Design review of the part built by this model. Coordinates are the model's own, in mm. A direction names the side the tool comes from. Coordinates: 2 decimals unless noted, no trailing zeros. Write each loop counter-clockwise with the first axis right and the second up, starting at its lowest first coordinate (ties: lowest second). Pieces come first, ordered by that corner, then holes. Notation, with made-up numbers: (-35, 1.25) -> (21, 1.25) arc R19 ccw to (21, 38.25) -> close; hole circle Ø6 at (-24, 42). An arc over 180 degrees is marked (long way). Write item = value, one per line. Start each with the question number.
```python
from build123d import *

# Parameters (mm, degrees)
SKETCH1_W                  = 30
SKETCH1_H                  = 30
SKETCH1_R                  = 1.6
SKETCH1_W_2                = 81.01
SKETCH1_H_2                = 12
BOSS_EXTRUDE1_DEPTH        = 6
SKETCH1_3_W                = 30
SKETCH1_3_H                = 30
SKETCH1_3_R                = 1.6
BOSS_EXTRUDE2_DEPTH        = 22.33
CUT_EXTRUDE1_DEPTH         = 88.671255266
SKETCH3_R                  = 2.55
CUT_EXTRUDE2_DEPTH         = 8
CUT_EXTRUDE3_DEPTH         = 4.5
SKETCH6_R                  = 5
CUT_EXTRUDE5_DEPTH         = 8.6
SKETCH7_R                  = 1.6
CUT_EXTRUDE6_DEPTH         = 112.183402538
SKETCH8_R                  = 2.85
CUT_EXTRUDE7_DEPTH         = 18
BOSS_EXTRUDE3_START        = 2.43
SKETCH9_R                  = 3.4
SKETCH9_R_2                = 2.55
BOSS_EXTRUDE3_DEPTH        = 2.43
CHAMFER1_SIZE              = 1.2
FILLET3_R                  = 4
CHAMFER2_SIZE              = 0.8
BOSS_EXTRUDE6_DEPTH        = 14
CUT_EXTRUDE10_REACH        = 116.661
SKETCH17_R                 = 1.1
FILLET5_R                  = 2
CUT_EXTRUDE11_DEPTH        = 3
CHAMFER3_SIZE              = 0.8
LPATTERN2_COUNT            = 3
LPATTERN2_PITCH            = 25
CHAMFER3_OF_LPATTERN2_SIZE = 0.8


with BuildPart() as part:
    # Sketch1 → Boss-Extrude1 (new body)
    # profile 1 of 2: a face of its own
    with BuildSketch(Plane.XY):
        with Locations((10, 10)):
            Rectangle(SKETCH1_W, SKETCH1_H)
        with Locations((20, 0)):
            Circle(SKETCH1_R, mode=Mode.SUBTRACT)
        with Locations((20, 20)):
            Circle(SKETCH1_R, mode=Mode.SUBTRACT)
        with Locations((0, 20)):
            Circle(SKETCH1_R, mode=Mode.SUBTRACT)
        Circle(SKETCH1_R, mode=Mode.SUBTRACT)
    # profile 2 of 2: a face of its own
    with BuildSketch(Plane.XY):
        with Locations((65.505, 10)):
            Rectangle(SKETCH1_W_2, SKETCH1_H_2)
    extrude(amount=BOSS_EXTRUDE1_DEPTH)

    # Sketch1<3> → Boss-Extrude2 (add)
    with BuildSketch(Plane.XY):
        with Locations((10, 10)):
            Rectangle(SKETCH1_3_W, SKETCH1_3_H)
        with Locations((20, 0)):
            Circle(SKETCH1_3_R, mode=Mode.SUBTRACT)
        with Locations((20, 20)):
            Circle(SKETCH1_3_R, mode=Mode.SUBTRACT)
        with Locations((0, 20)):
            Circle(SKETCH1_3_R, mode=Mode.SUBTRACT)
        Circle(SKETCH1_3_R, mode=Mode.SUBTRACT)
    extrude(amount=BOSS_EXTRUDE2_DEPTH)

    # Sketch2 → Cut-Extrude1 (cut, through all)
    with BuildSketch(Plane(origin=(25, 0, 0), x_dir=(0, 0, -1), z_dir=(1, 0, 0))):
        with BuildLine():
            Line((-6.54075, 16.488632043), (-9.2445, 16.488632043))
            Line((-9.2445, 16.488632043), (-10.381879417, 16.288081364))
            ThreePointArc((-10.381879417, 16.288081364), (-11.49719937, 14.886920062), (-13.024482689, 15.822119108))
            Line((-13.024482689, 15.822119108), (-14.11125, 15.630492709))
            Line((-14.11125, 15.630492709), (-14.11125, 4.368771376))
            Line((-14.11125, 4.368771376), (-13.024482689, 4.177144977))
            ThreePointArc((-13.024482689, 4.177144977), (-11.49719937, 5.112344024), (-10.381879417, 3.711182721))
            Line((-10.381879417, 3.711182721), (-9.2445, 3.510632043))
            Line((-9.2445, 3.510632043), (-6.54075, 3.510632043))
            Line((-6.54075, 3.510632043), (-6, 4.051382043))
            Line((-6, 4.051382043), (-6, 15.947882043))
            Line((-6, 15.947882043), (-6.54075, 16.488632043))
        make_face()
    extrude(amount=-CUT_EXTRUDE1_DEPTH, mode=Mode.SUBTRACT)

    # Sketch3 → Cut-Extrude2 (cut)
    with BuildSketch(Plane.XY.offset(22.33)):
        with Locations((10, 10)):
            Circle(SKETCH3_R)
    extrude(amount=-CUT_EXTRUDE2_DEPTH, mode=Mode.SUBTRACT)

    # Sketch5 → Cut-Extrude3 (cut)
    with BuildSketch(Plane(origin=(0, 0, 14.11125), x_dir=(-1, 0, 0), z_dir=(0, 0, -1))):
        Polygon((-5.32346282, 10), (-7.66173141, 14.05), (-12.33826859, 14.05), (-14.67653718, 10), (-12.33826859, 5.95), (-7.66173141, 5.95), align=None)
    extrude(amount=-CUT_EXTRUDE3_DEPTH, mode=Mode.SUBTRACT)

    # Sketch6 → Cut-Extrude5 (cut)
    with BuildSketch(Plane(origin=(0, 0, 0), x_dir=(-1, 0, 0), z_dir=(0, 0, -1))):
        with Locations((-10, 10)):
            Circle(SKETCH6_R)
    extrude(amount=-CUT_EXTRUDE5_DEPTH, mode=Mode.SUBTRACT)

    # Sketch7 → Cut-Extrude6 (cut, through all)
    with BuildSketch(Plane(origin=(0, 0, 0), x_dir=(-1, 0, 0), z_dir=(0, 0, -1))):
        with BuildLine():
            ThreePointArc((-101.1, 10), (-99.5, 8.4), (-97.9, 10))
            Line((-97.9, 10), (-101.1, 10))
        make_face()
        with BuildLine():
            Line((-101.1, 10), (-97.9, 10))
            ThreePointArc((-97.9, 10), (-99.5, 11.6), (-101.1, 10))
        make_face()
        with Locations((-74.5, 10)):
            Circle(SKETCH7_R)
        with Locations((-49.5, 10)):
            Circle(SKETCH7_R)
    extrude(amount=-CUT_EXTRUDE6_DEPTH, mode=Mode.SUBTRACT)

    # Sketch8 → Cut-Extrude7 (cut)
    with BuildSketch(Plane.XY.offset(22.33)):
        with Locations((20, 20)):
            Circle(SKETCH8_R)
        with Locations((20, 0)):
            Circle(SKETCH8_R)
        Circle(SKETCH8_R)
        with Locations((0, 20)):
            Circle(SKETCH8_R)
    extrude(amount=-CUT_EXTRUDE7_DEPTH, mode=Mode.SUBTRACT)

    # Sketch9 → Boss-Extrude3 (add)
    with BuildSketch(Plane.XY.offset(22.33).offset(BOSS_EXTRUDE3_START)):
        with Locations(Location((10, 10, 0), (0, 0, 180))):
            Circle(SKETCH9_R)
        with Locations((10, 10)):
            Circle(SKETCH9_R_2, mode=Mode.SUBTRACT)
    extrude(amount=-BOSS_EXTRUDE3_DEPTH)

    # Chamfer1
    chamfer1_edges = [part.edges().sort_by_distance(p)[0] for p in [
        (13.4, 10, 22.33),
    ]]
    chamfer(chamfer1_edges, length=CHAMFER1_SIZE)

    # Fillet3
    fillet3_edges = [part.edges().sort_by_distance(p)[0] for p in [
        (-5, -5, 11.165),
        (-5, 25, 11.165),
        (25, 25, 11.165),
        (25, 16, 3),
        (106.01, 16, 3),
        (106.01, 4, 3),
        (25, 4, 3),
        (25, -5, 11.165),
    ]]
    fillet(fillet3_edges, radius=FILLET3_R)

    # Chamfer2
    chamfer2_edges = [part.edges().sort_by_distance(p)[0] for p in [
        (-2.85, 20, 22.33),
        (-2.85, 0, 22.33),
        (17.15, 0, 22.33),
        (17.15, 20, 22.33),
    ]]
    chamfer(chamfer2_edges, length=CHAMFER2_SIZE)

    # Sketch15 → Boss-Extrude6 (add)
    with BuildSketch(Plane.XY.offset(22.33)):
        Polygon((18.343145751, 31), (12.343145751, 25), (18, 25), (21, 28), (27, 28), (27, 31), align=None)
    extrude(amount=-BOSS_EXTRUDE6_DEPTH)

    # Sketch17 → Cut-Extrude10 (cut, up to next)
    with BuildSketch(Plane(origin=(0, 31, 0), x_dir=(1, 0, 0), z_dir=(0, 1, 0)), mode=Mode.PRIVATE) as cut_extrude10_sk1:
        with Locations(Location((24, -11.33, 0), (0, 0, 180))):
            Circle(SKETCH17_R)
    cut_extrude10_tool1 = extrude(cut_extrude10_sk1.sketch, amount=-CUT_EXTRUDE10_REACH, mode=Mode.PRIVATE) & part.part
    # Sketch17 → Cut-Extrude10 (cut, up to next)
    with BuildSketch(Plane(origin=(0, 31, 0), x_dir=(1, 0, 0), z_dir=(0, 1, 0)), mode=Mode.PRIVATE) as cut_extrude10_sk2:
        with Locations(Location((24, -17.83, 0), (0, 0, 180))):
            Circle(SKETCH17_R)
    cut_extrude10_tool2 = extrude(cut_extrude10_sk2.sketch, amount=-CUT_EXTRUDE10_REACH, mode=Mode.PRIVATE) & part.part
    add(cut_extrude10_tool1.solids().sort_by_distance((24, 31, 11.33))[0], mode=Mode.SUBTRACT)
    add(cut_extrude10_tool2.solids().sort_by_distance((24, 31, 17.83))[0], mode=Mode.SUBTRACT)

    # Fillet5
    # the kernel refuses this fillet: 2 mm, written as the material it adds along each edge
    with BuildSketch(Plane(origin=(21, 28, 22.33), x_dir=(-0.7071067811865475, -0.7071067811865475, 0), z_dir=(0, 0, -1))) as fillet5_piece_1:
        with BuildLine():
            CenterArc((FILLET5_R * 0.414213562373, -FILLET5_R), FILLET5_R, 90, 45)
            Line((-FILLET5_R * 0.292893218813, -FILLET5_R * 0.292893218813), (0, 0))
            Line((0, 0), (FILLET5_R * 0.414213562373, 0))
        make_face()
    extrude(amount=14)
    with BuildSketch(Plane(origin=(12.343145751, 25, 22.33), x_dir=(-1, 0, 0), z_dir=(0, 0, -1))) as fillet5_piece_2:
        with BuildLine():
            CenterArc((FILLET5_R * 0.414213562373, FILLET5_R), FILLET5_R, 225, 45)
            Line((-FILLET5_R * 0.292893218813, FILLET5_R * 0.292893218813), (0, 0))
            Line((0, 0), (FILLET5_R * 0.414213562373, 0))
        make_face()
    extrude(amount=14)
    with BuildSketch(Plane(origin=(18, 25, 22.33), x_dir=(0.9993539414176275, -0.03594022500003582, 0), z_dir=(0, 0, -1))) as fillet5_piece_3:
        with BuildLine():
            CenterArc((4.541773641, -1.944797545), FILLET5_R, 103.492916805, 119.447416414)
            Line((3.07764659, -3.307270289), (2.931233885, -3.443517564))
            Line((2.931233885, -3.443517564), (-0.146412705, -0.136247274))
            Line((-0.146412705, -0.136247274), (0.007188045, 0.199870788))
            ThreePointArc((0.007188045, 0.199870788), (3.005249869, 0.092050113), (4.028458305, 0.194479755))
            Line((4.028458305, 0.194479755), (4.075123335, 0))
        make_face()
    extrude(amount=14)
    # the kernel refuses this fillet: 2 mm, written as the material it takes off along each edge
    with BuildSketch(Plane(origin=(27, 23, 22.33), x_dir=(-1, 0, 0), z_dir=(0, 1, 0))) as fillet5_2_piece_1:
        with BuildLine():
            CenterArc((FILLET5_R, -FILLET5_R), FILLET5_R, 90, 90)
            Line((0, -FILLET5_R), (0, 0))
            Line((0, 0), (FILLET5_R, 0))
        make_face()
    extrude(amount=13, mode=Mode.SUBTRACT)
    with BuildSketch(Plane(origin=(27, 23, 8.33), x_dir=(-1, 0, 0), z_dir=(0, 1, 0))) as fillet5_2_piece_2:
        with BuildLine():
            CenterArc((FILLET5_R, FILLET5_R), FILLET5_R, 180, 90)
            Line((0, FILLET5_R), (0, 0))
            Line((0, 0), (FILLET5_R, 0))
        make_face()
    extrude(amount=13, mode=Mode.SUBTRACT)
    with BuildSketch(Plane(origin=(18.343145751, 31, 24.401067812), x_dir=(-0.7071067811865476, -0.7071067811865476, 0), z_dir=(0, 0, -1))) as fillet5_2_piece_3:
        with BuildLine():
            CenterArc((FILLET5_R * 0.414213562373, -FILLET5_R), FILLET5_R, 90, 45)
            Line((-FILLET5_R * 0.292893218813, -FILLET5_R * 0.292893218813), (0, 0))
            Line((0, 0), (FILLET5_R * 0.414213562373, 0))
        make_face()
    extrude(amount=18.142135624, mode=Mode.SUBTRACT)

    # Sketch10 → Cut-Extrude11 (cut)
    with BuildSketch(Plane(origin=(0, 0, 0), x_dir=(-1, 0, 0), z_dir=(0, 0, -1))):
        Polygon((-97.883419246, 12.8), (-101.116580754, 12.8), (-102.733161507, 10), (-101.116580754, 7.2), (-97.883419246, 7.2), (-96.266838493, 10), align=None)
    cut_extrude11 = extrude(amount=-CUT_EXTRUDE11_DEPTH, mode=Mode.SUBTRACT)

    # Chamfer3
    chamfer3_edges = [part.edges().sort_by_distance(p)[0] for p in [
        (97.075128869, 11.4, 0),
        (99.5, 12.8, 0),
        (101.924871131, 11.4, 0),
        (101.924871131, 8.6, 0),
        (99.5, 7.2, 0),
        (97.075128869, 8.6, 0),
    ]]
    chamfer(chamfer3_edges, length=CHAMFER3_SIZE)

    # LPattern2: Cut-Extrude11 ×3
    with Locations(*[(-i * LPATTERN2_PITCH, 0, 0) for i in range(1, LPATTERN2_COUNT)]):
        add(cut_extrude11, mode=Mode.SUBTRACT)

    # Chamfer3 of LPattern2
    chamfer3_of_lpattern2_edges = [part.edges().sort_by_distance(p)[0] for p in [
        (72.075128869, 11.4, 0),
        (74.5, 12.8, 0),
        (76.924871131, 11.4, 0),
        (76.924871131, 8.6, 0),
        (74.5, 7.2, 0),
        (72.075128869, 8.6, 0),
        (47.075128869, 11.4, 0),
        (49.5, 12.8, 0),
        (51.924871131, 11.4, 0),
        (51.924871131, 8.6, 0),
        (49.5, 7.2, 0),
        (47.075128869, 8.6, 0),
    ]]
    chamfer(chamfer3_of_lpattern2_edges, length=CHAMFER3_OF_LPATTERN2_SIZE)


solid = part.part
```
(1) For pin 1 Ø1.1 at (x, z) = (50, 2) entering from -Y; pin 2 Ø5 at (x, y) = (65, 0.5) entering from +Z; pin 3 Ø11 at (x, z) = (6, 10) entering from +Y; pin 4 Ø12 at (y, z) = (18.5, 9) entering from +X, all flat-tipped, find the tip position at first contact; note any pin that passes through.
(2) For faces 4 (the face through (97.086, 8.58, 1.885)), 5 (the face through (0, -2, 4.33)), 6 (the face through (23.797, -3.859, 11.321)), list the 3-axis set-ups (+Z, -Z, +X, -X, +Y, -Y) from which the entire face can be reached by the end or side of a thin tool; tool diameter is ignored.
(3) Take a section at D-D, the plane x = 38.5. State the section outline as (y, z) points, then the cut area to 3 significant figures.
(4) Take a section at C-C, the plane x = 99.5. State the section outline as (y, z) points, then the cut area to 3 significant figures.
(5) For line 1 (X direction, y = 20, z = 1.8); line 2 (Z direction, x = 24, y = 30.05), list the stretches that pass through material, from the lowest coordinate up.
(6) Take a section at B-B, the plane z = 15.25. State the section outline as (x, y) points.
(7) Mouldability with a two-part tool opening along Y and no side actions: class faces 1 (the face through (10, 5, 22.33)), 2 (the face through (6.48, 12, 16.33)), 3 (the face through (8.4, 13, 24.2)) as pulls with the +Y half, pulls with the -Y half, needs draft (parallel to the pull), parting line crosses it, or undercut.
Report:
q1.pin_1 = 4
q1.pin_2 = through
q1.pin_3 = 25
q1.pin_4 = 105.79
q2.face_4 = -Z
q2.face_5 = +Z
q2.face_6 = +Z, -Z, +X, -Y
q3.outline = (4, 0) -> (16, 0) -> (16, 6) -> (4, 6) -> close
q3.area = 72.0 mm2
q4.outline = (4, 0) -> (6.4, 0) -> (7.2, 0.8) -> (7.2, 3) -> (8.4, 3) -> (8.4, 6) -> (4, 6) -> close; (11.6, 3) -> (12.8, 3) -> (12.8, 0.8) -> (13.6, 0) -> (16, 0) -> (16, 6) -> (11.6, 6) -> close
q4.area = 45.0 mm2
q5.line_1 = -5 to -1.6, 1.6 to 18.4, 21.6 to 25
q5.line_2 = 8.33 to 10.23, 12.43 to 16.73, 18.93 to 22.33
q6.outline = (-5, -1) arc R4 ccw to (-1, -5) -> (21, -5) arc R4 ccw to (25, -1) -> (25, 21) arc R4 ccw to (22.07, 24.85) arc R2 cw to (20.86, 27.75) arc R2 cw to (21.83, 28) -> (27, 28) -> (27, 31) -> (19.17, 31) arc R2 ccw to (17.76, 30.41) -> (12.93, 25.59) arc R2 cw to (11.51, 25) -> (-1, 25) arc R4 ccw to (-5, 21) -> close; hole circle Ø5.7 at (0, 0); hole circle Ø5.7 at (0, 20); hole (5.32, 10) -> (7.66, 5.95) -> (12.34, 5.95) -> (14.68, 10) -> (12.34, 14.05) -> (7.66, 14.05) -> close; hole circle Ø5.7 at (20, 0); hole circle Ø5.7 at (20, 20)
q7.face_1 = needs draft
q7.face_2 = undercut
q7.face_3 = parting line crosses it
